from build123d import *

# Parameters (mm, degrees)
SKETCH002_R      = 115
PAD001_DEPTH     = 8.7
SKETCH005_W      = 5.7
SKETCH005_H      = 185.2
POCKET_DEPTH     = 257
SKETCH016_W      = 13
SKETCH016_H      = 6
POCKET004_DEPTH  = 5
CHAMFER001_ANGLE = 47
CHAMFER001_SIZE  = 4.6
SKETCH018_R      = 2.1
POCKET005_DEPTH  = 10
SKETCH019_R      = 2.1
POCKET006_DEPTH  = 10
POCKET007_DEPTH  = 5


with BuildPart() as part:
    # Sketch002 → Pad001 (new body)
    with BuildSketch(Plane.XY):
        Circle(SKETCH002_R)
    extrude(amount=PAD001_DEPTH)

    # Sketch005 (on DatumPlane) → Pocket (cut)
    with BuildSketch(Plane(origin=(115, 0, 4.35), x_dir=(0, 0, -1), z_dir=(1, 0, 0))):
        with Locations((-1.5, 0)):
            Rectangle(SKETCH005_W, SKETCH005_H)
    extrude(amount=-POCKET_DEPTH, mode=Mode.SUBTRACT)

    # Sketch016 (on Face6 of Pocket) → Pocket004 (cut)
    with BuildSketch(Plane.XZ.offset(-92.6)):
        with Locations((-61.897977, 6)):
            Rectangle(SKETCH016_W, SKETCH016_H)
    extrude(amount=-POCKET004_DEPTH, mode=Mode.SUBTRACT)

    # Chamfer001
    chamfer001_edges = [part.edges().sort_by_distance(p)[0] for p in [
        (-55.397977, 92.6, 5.85),
    ]]
    chamfer001_side = part.faces().sort_by_distance((6.397346, 92.6, 5.85))[0]
    chamfer(chamfer001_edges, length=CHAMFER001_SIZE, angle=CHAMFER001_ANGLE, reference=chamfer001_side)

    # Sketch018 (on Face1 of Chamfer001) → Pocket005 (cut)
    with BuildSketch(Plane.XY.offset(8.7)):
        with Locations((15.447874, 97.534228)):
            Circle(SKETCH018_R)
        with Locations((-15.447903, 97.534224)):
            Circle(SKETCH018_R)
    extrude(amount=-POCKET005_DEPTH, mode=Mode.SUBTRACT)

    # Sketch019 (on Face11 of Pocket005) → Pocket006 (cut)
    with BuildSketch(Plane.XY.offset(8.7)):
        with Locations((-15.447907, -97.534223)):
            Circle(SKETCH019_R)
        with Locations((15.447907, -97.534223)):
            Circle(SKETCH019_R)
    extrude(amount=-POCKET006_DEPTH, mode=Mode.SUBTRACT)

    # Sketch020 (on Face12 of Pocket006) → Pocket007 (cut)
    with BuildSketch(Plane(origin=(0, 0, 0), x_dir=(1, 0, 0), z_dir=(0, 0, -1))):
        Polygon((14.79085, 93.385937), (18.711887, 94.891084), (19.368911, 99.039375), (16.104897, 101.68252), (12.18386, 100.177373), (11.526836, 96.029082), align=None)
        Polygon((14.790851, -93.385937), (18.711888, -94.891084), (19.368912, -99.039375), (16.104898, -101.682519), (12.183861, -100.177373), (11.526837, -96.029082), align=None)
        Polygon((-14.79085, 93.385937), (-18.711887, 94.891084), (-19.368911, 99.039375), (-16.104897, 101.68252), (-12.18386, 100.177373), (-11.526836, 96.029082), align=None)
        Polygon((-14.790851, -93.385937), (-18.711888, -94.891084), (-19.368912, -99.039375), (-16.104898, -101.682519), (-12.183861, -100.177373), (-11.526837, -96.029082), align=None)
    extrude(amount=-POCKET007_DEPTH, mode=Mode.SUBTRACT)


solid = part.part
Geometry check sheet. Reference: the model listing, model coordinates, mm. A direction names the side the tool comes from. Give positions to 0.01 mm unless a question says otherwise; leave off trailing zeros. Loops run counter-clockwise (first coordinate to the right, second up) from the corner with the lowest first, then second, coordinate; pieces in that order, holes last. Notation, with made-up numbers: (56, -29) -> (65, -29) arc R6 ccw to (65, -24) -> close; hole circle Ø8 at (26.5, 58.5). An arc over 180 degrees is marked (long way). Answer in a Markdown table with one row per item. Add a question column.
1) Set-up check for faces 4 (the face through (17.1, -99.4, 5)), 5 (the face through (10, 92.6, 6)), 6 (the face through (-1, -101, 8.7)), 7 (the face through (-2, 2, 0)), 8 (the face through (-58, 97.6, 6)): record each of +Z, -Z, +X, -X, +Y, -Y from which the full face is reachable in a straight line by a thin tool's end or side.
2) Cross-section at D-D on x = 63. Record the boundary of the cut face in (y, z).
3) Cross-section at C-C on y = 0. Record the boundary of the cut face in (x, z), and give its area (3 significant figures).
4) Gauge pin test, flat ends, axial feed: P1, Ø10, axis at x = -23.5, y = 10.5, coming from the +Z side; P2, Ø2.5, axis at x = -57, z = 6, coming from the -Y side; P3, Ø4, axis at x = -15.45, y = 97.53, coming from the +Z side; P4, Ø6.5, axis at x = 13.5, y = 96, coming from the -Z side. Record the tip position at first contact, or that the pin passes through.
5) Draft check along X on faces 1 (the face through (-17.1, -99.4, 5)), 2 (the face through (-53.13, 95.1, 5.81)), 3 (the face through (2, 1, 3)). Enter one of: pulls with the +X half, pulls with the -X half, needs draft (parallel to the pull), parting line crosses it, or undercut.
6) Cross-section at A-A on z = 1.5. Record the boundary of the cut face in (x, y).
7) Material ranges on probe 1 along Y at (x, z) = (-18, 1.5); probe 2 along Z at (x, y) = (50.5, 41.5); probe 3 along Y at (x, z) = (-15, 6.5), recorded low to high. Write a range as from..to.
8) Cross-section at B-B on x = 0. Record the boundary of the cut face in (y, z), and give its area (3 significant figures).
Outcome:
| question | item | result |
|---|---|---|
| 1 | face 4 | -Z |
| 1 | face 5 | +Z, +X, -X |
| 1 | face 6 | +Z, +X, -X, +Y, -Y |
| 1 | face 7 | -Z, +X, -X, +Y, -Y |
| 1 | face 8 | +Z, -X |
| 2 | outline | (-96.21, 0) -> (96.21, 0) -> (96.21, 8.7) -> (92.6, 8.7) -> (92.6, 3) -> (-92.6, 3) -> (-92.6, 8.7) -> (-96.21, 8.7) -> close |
| 3 | outline | (-115, 0) -> (115, 0) -> (115, 3) -> (-115, 3) -> close |
| 3 | area | 690 mm^2 |
| 4 | P1 | stops at z = 3 |
| 4 | P2 | stops at y = -100.58 |
| 4 | P3 | passes through |
| 4 | P4 | stops at z = 0 |
| 5 | face 1 | undercut |
| 5 | face 2 | pulls with the -X half |
| 5 | face 3 | needs draft |
| 6 | outline | circle Ø230 at (0, 0); hole (-19.37, -99.04) -> (-16.1, -101.68) -> (-12.18, -100.18) -> (-11.53, -96.03) -> (-14.79, -93.39) -> (-18.71, -94.89) -> close; hole (-19.37, 99.04) -> (-18.71, 94.89) -> (-14.79, 93.39) -> (-11.53, 96.03) -> (-12.18, 100.18) -> (-16.1, 101.68) -> close; hole (11.53, -96.03) -> (12.18, -100.18) -> (16.1, -101.68) -> (19.37, -99.04) -> (18.71, -94.89) -> (14.79, -93.39) -> close; hole (11.53, 96.03) -> (14.79, 93.39) -> (18.71, 94.89) -> (19.37, 99.04) -> (16.1, 101.68) -> (12.18, 100.18) -> close |
| 7 | probe 1 | y = -113.58..-100.15, -94.62..94.62, 100.15..113.58 |
| 7 | probe 2 | z = 0..3 |
| 7 | probe 3 | y = -114.02..-99.59, -95.48..-92.6, 92.6..95.48, 99.59..114.02 |
| 8 | outline | (-115, 0) -> (115, 0) -> (115, 8.7) -> (92.6, 8.7) -> (92.6, 3) -> (-92.6, 3) -> (-92.6, 8.7) -> (-115, 8.7) -> close |
| 8 | area | 945 mm^2 |
